```python
from build123d import *

# Parameters (mm, degrees)
SKETCH_W            = 175
SKETCH_H            = 140
SKETCH_R            = 2.2
PAD_DEPTH           = 3
SKETCH001_W         = 175
SKETCH001_H         = 10
PAD001_DEPTH        = 14
SKETCH002_R         = 2.2
POCKET_DEPTH        = 140.001
SKETCH003_W         = 7.2
SKETCH003_H         = 3.5
POCKET001_DEPTH     = 11.2
LINEARPATTERN_COUNT = 7
LINEARPATTERN_PITCH = 25.436
POCKET002_DEPTH     = 0.5
PAD002_DEPTH        = 12.7
POCKET003_DEPTH     = 3.001
SKETCH007_R         = 4.5
PAD003_DEPTH        = 12.7
SKETCH008_R         = 1.5
POCKET004_DEPTH     = 14
CHAMFER_SIZE        = 0.75


with BuildPart() as part:
    # Sketch → Pad (new body)
    with BuildSketch(Plane.XY):
        with Locations((0, 70)):
            Rectangle(SKETCH_W, SKETCH_H)
        with Locations((-79.5, 115)):
            Circle(SKETCH_R, mode=Mode.SUBTRACT)
        with Locations((79.5, 115)):
            Circle(SKETCH_R, mode=Mode.SUBTRACT)
        with Locations((79.5, 25)):
            Circle(SKETCH_R, mode=Mode.SUBTRACT)
        with Locations((-79.5, 25)):
            Circle(SKETCH_R, mode=Mode.SUBTRACT)
        with Locations((-75, 10.5)):
            Circle(SKETCH_R, mode=Mode.SUBTRACT)
        with Locations((-25, 10.5)):
            Circle(SKETCH_R, mode=Mode.SUBTRACT)
        with Locations((25, 10.5)):
            Circle(SKETCH_R, mode=Mode.SUBTRACT)
        with Locations((75, 10.5)):
            Circle(SKETCH_R, mode=Mode.SUBTRACT)
    extrude(amount=PAD_DEPTH)

    # Sketch001 (on Face14 of Pad) → Pad001 (join)
    with BuildSketch(Plane.XY.offset(3)):
        with Locations((0, 135)):
            Rectangle(SKETCH001_W, SKETCH001_H)
    extrude(amount=PAD001_DEPTH)

    # Sketch002 (on Face5 of Pad001) → Pocket (cut, through all)
    with BuildSketch(Plane(origin=(0, 140, 0), x_dir=(-1, 0, 0), z_dir=(0, 1, 0))):
        with Locations((-75.508, 10)):
            Circle(SKETCH002_R)
        with Locations((-50.072, 10)):
            Circle(SKETCH002_R)
        with Locations((-24.636, 10)):
            Circle(SKETCH002_R)
        with Locations((0.8, 10)):
            Circle(SKETCH002_R)
        with Locations((26.236, 10)):
            Circle(SKETCH002_R)
        with Locations((51.672, 10)):
            Circle(SKETCH002_R)
        with Locations((77.108, 10)):
            Circle(SKETCH002_R)
    extrude(amount=-POCKET_DEPTH, mode=Mode.SUBTRACT)

    # Sketch003 (on Face18 of Pocket) → Pocket001 (cut)
    with BuildSketch(Plane.XY.offset(17)):
        with Locations((75.508, 135)):
            Rectangle(SKETCH003_W, SKETCH003_H)
    pocket001 = extrude(amount=-POCKET001_DEPTH, mode=Mode.SUBTRACT)

    # LinearPattern: Pocket001 ×7
    with Locations(*[(-i * LINEARPATTERN_PITCH, 0, 0) for i in range(1, LINEARPATTERN_COUNT)]):
        add(pocket001, mode=Mode.SUBTRACT)

    # Sketch004 (on Face7 of LinearPattern) → Pocket002 (cut)
    with BuildSketch(Plane.XY.offset(3)):
        Polygon((84, 68.55), (84, 61.45), (82.3, 61.45), (82.3, 64.15), (76.3, 64.15), (76.3, 65.85), (82.3, 65.85), (82.3, 68.55), align=None)
    extrude(amount=-POCKET002_DEPTH, mode=Mode.SUBTRACT)

    # Sketch005 (on Face7 of Pocket002) → Pad002 (join)
    with BuildSketch(Plane.XY.offset(3)):
        with BuildLine():
            ThreePointArc((65, 103), (67, 105), (65, 107))
            Line((65, 107), (-65, 107))
            ThreePointArc((-65, 107), (-67, 105), (-65, 103))
            Line((65, 103), (-65, 103))
        make_face()
    extrude(amount=PAD002_DEPTH)

    # Sketch006 (on Face7 of Pad002) → Pocket003 (cut, through all)
    with BuildSketch(Plane.XY.offset(3)):
        with BuildLine():
            Line((-57.5, 98), (57.5, 98))
            ThreePointArc((62.5, 93), (61.0355339059, 96.5355339059), (57.5, 98))
            Line((62.5, 93), (62.5, 25))
            ThreePointArc((57.5, 20), (61.0355339059, 21.4644660941), (62.5, 25))
            Line((57.5, 20), (-57.5, 20))
            ThreePointArc((-62.5, 25), (-61.0355339059, 21.4644660941), (-57.5, 20))
            Line((-62.5, 25), (-62.5, 93))
            ThreePointArc((-57.5, 98), (-61.0355339059, 96.5355339059), (-62.5, 93))
        make_face()
    extrude(amount=-POCKET003_DEPTH, mode=Mode.SUBTRACT)

    # Sketch007 (on Face7 of Pocket003) → Pad003 (join)
    with BuildSketch(Plane.XY.offset(3)):
        with Locations((72.5, 79)):
            Circle(SKETCH007_R)
        with Locations((72.5, 39)):
            Circle(SKETCH007_R)
    extrude(amount=PAD003_DEPTH)

    # Sketch008 (on Face4 of Pad003) → Pocket004 (cut)
    with BuildSketch(Plane(origin=(0, 0, 0), x_dir=(1, 0, 0), z_dir=(0, 0, -1))):
        with Locations((72.5, -79)):
            Circle(SKETCH008_R)
        with Locations((72.5, -39)):
            Circle(SKETCH008_R)
    extrude(amount=-POCKET004_DEPTH, mode=Mode.SUBTRACT)

    # Chamfer
    chamfer_edges = [part.edges().sort_by_distance(p)[0] for p in [
        (0, 140, 0),
        (-87.5, 70, 0),
        (87.5, 70, 0),
        (0, 0, 0),
        (-77.2, 10.5, 0),
        (-27.2, 10.5, 0),
        (71, 39, 0),
        (72.8, 10.5, 0),
        (71, 79, 0),
        (22.8, 10.5, 0),
        (61.035534, 96.535534, 0),
        (62.5, 59, 0),
        (0, 98, 0),
        (61.035534, 21.464466, 0),
        (-61.035534, 96.535534, 0),
        (0, 20, 0),
        (-62.5, 59, 0),
        (-61.035534, 21.464466, 0),
        (77.3, 115, 0),
        (77.3, 25, 0),
        (-81.7, 115, 0),
        (-81.7, 25, 0),
    ]]
    chamfer(chamfer_edges, length=CHAMFER_SIZE)


solid = part.part
```
For this review, take the finished solid that the model builds, in its own axes (mm). A direction names the side the tool comes from. Coordinates: 2 decimals unless noted, no trailing zeros. Loops run counter-clockwise (first coordinate to the right, second up) from the corner with the lowest first, then second, coordinate; pieces in that order, holes last. Notation, with made-up numbers: (55, -35) - (69, -35) arc R25 ccw to (69, -9) - close; hole circle Ø5 at (-36.75, 23). An arc over 180 degrees is marked (long way). Use one line per item in the form item = value. Start each with the question number.
1) For pin 1 (5 mm diameter, centred on y = 39, z = 12, fed in from +X); pin 2 (2 mm diameter, centred on x = 0.5, z = 9.5, fed in from -Y); pin 3 (2 mm diameter, centred on x = 79, y = 66, fed in from +Z); pin 4 (5 mm diameter, centred on x = 58, y = 90.5, fed in from +Z), all flat-tipped, find the tip position at first contact; note any pin that passes through.
2) To check wall thickness, follow probe 1 along Y at (x, z) = (72.5, 5.75); probe 2 along Y at (x, z) = (72.5, 9.25); probe 3 along Y at (x, z) = (-3.5, 15.25). State the ranges of each line that lie inside material, in increasing order. Write a range as from..to.
3) Take a section at A-A (x = 8). State the section outline as (y, z) points.
4) For faces 4 (the face through (-4.4, 135, 11)), 5 (the face through (80.683, 116.855, 1.859)), 6 (the face through (72, 79, 15.7)), 7 (the face through (51.69, 131.65, 11.49)), list the 3-axis set-ups (+Z, -Z, +X, -X, +Y, -Y) from which the entire face can be reached by the end or side of a thin tool; tool diameter is ignored.
5) Draft analysis for pull direction X (two halves, no side actions). For faces 1 (the face through (73.41, 138.4, 10.66)), 2 (the face through (-27.419, 131.648, 11.855)), 3 (the face through (-1, 140, 7)), state which applies: released by +X, released by -X, zero draft, split by the parting line, or undercut.
From the geometry:
q1.pin_1 = 77
q1.pin_2 = 103
q1.pin_3 = 3
q1.pin_4 = through
q2.probe_1 = 34.5..37.5, 40.5..43.5, 74.5..77.5, 80.5..83.5, 130..140
q2.probe_2 = 34.5..37.5, 40.5..43.5, 74.5..77.5, 80.5..83.5, 130..133.25, 136.75..140
q2.probe_3 = 103..107, 130..133.25, 136.75..140
q3.outline = (0, 0.75) - (0.75, 0) - (19.25, 0) - (20, 0.75) - (20, 3) - (0, 3) - close; (98, 0.75) - (98.75, 0) - (139.25, 0) - (140, 0.75) - (140, 17) - (130, 17) - (130, 3) - (107, 3) - (107, 15.7) - (103, 15.7) - (103, 3) - (98, 3) - close
q4.face_4 = +Z
q4.face_5 = +Z, -Z
q4.face_6 = +Z, +X, -X, -Y
q4.face_7 = +Y
q5.face_1 = undercut
q5.face_2 = undercut
q5.face_3 = zero draft
